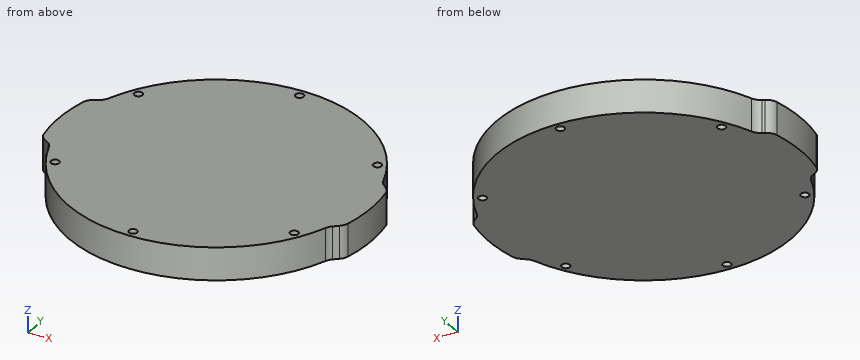
from build123d import *

# Parameters (mm, degrees)
SKETCH1_R           = 1.6
BOSS_EXTRUDE1_DEPTH = 12.7
FILLET1_R           = 5


with BuildPart() as part:
    # Sketch1 → Boss-Extrude1 (new body)
    with BuildSketch(Plane.XY):
        with BuildLine():
            Line((-59.281721466, 15), (-54.404710274, 17.5))
            ThreePointArc((-54.404710274, 17.5), (0, 57.15), (54.404710274, 17.5))
            Line((54.404710274, 17.5), (58.525108251, 13.886475587))
            ThreePointArc((58.525108251, 13.886475587), (60.15, 0), (58.525108251, -13.886475587))
            Line((58.525108251, -13.886475587), (54.404710274, -17.5))
            ThreePointArc((54.404710274, -17.5), (0, -57.15), (-54.404710274, -17.5))
            Line((-54.404710274, -17.5), (-59.281721466, -15))
            ThreePointArc((-59.281721466, -15), (-61.15, 0), (-59.281721466, 15))
        make_face()
        with Locations((0, 53.975)):
            Circle(SKETCH1_R, mode=Mode.SUBTRACT)
        with Locations((46.743721169, 26.9875)):
            Circle(SKETCH1_R, mode=Mode.SUBTRACT)
        with Locations((46.743721169, -26.9875)):
            Circle(SKETCH1_R, mode=Mode.SUBTRACT)
        with Locations((0, -53.975)):
            Circle(SKETCH1_R, mode=Mode.SUBTRACT)
        with Locations((-46.743721169, -26.9875)):
            Circle(SKETCH1_R, mode=Mode.SUBTRACT)
        with Locations((-46.743721169, 26.9875)):
            Circle(SKETCH1_R, mode=Mode.SUBTRACT)
    extrude(amount=BOSS_EXTRUDE1_DEPTH)

    # Fillet1
    fillet1_edges = [part.edges().sort_by_distance(p)[0] for p in [
        (58.525108251, -13.886475587, 6.35),
        (54.404710274, -17.5, 6.35),
        (-54.404710274, -17.5, 6.35),
        (-59.281721466, -15, 6.35),
        (-59.281721466, 15, 6.35),
        (-54.404710274, 17.5, 6.35),
        (54.404710274, 17.5, 6.35),
        (58.525108251, 13.886475587, 6.35),
    ]]
    fillet(fillet1_edges, radius=FILLET1_R)


solid = part.part
Read the model definition and answer for the solid it produces. Units are mm, in the model's axes. Coordinates: 2 decimals unless noted, no trailing zeros. Write each loop counter-clockwise with the first axis right and the second up, starting at its lowest first coordinate (ties: lowest second). Pieces come first, ordered by that corner, then holes. Notation, with made-up numbers: M 72,7.25 L 115,7.25 A8 cw 115,22.25 Z; hole C -23,86 d10. An arc over 180 degrees is marked long. Use a Markdown table: item, result.
Q1. The part is cut by section A-A, the plane x = 0. Write down the section's boundary in (y, z) (3 decimals).
Answer block:
| item | result |
|---|---|
| outline | M -57.15,0 L -55.575,0 L -55.575,12.7 L -57.15,12.7 Z; M -52.375,0 L 52.375,0 L 52.375,12.7 L -52.375,12.7 Z; M 55.575,0 L 57.15,0 L 57.15,12.7 L 55.575,12.7 Z |
Q2. The part is cut by section B-B, the plane z = 6.75. Give the number of separate pieces and of enclosed holes in the cut face, then the cut area to 3 significant figures.
Answer block:
| item | result |
|---|---|
| separate pieces | 1 |
| enclosed holes | 6 |
| area | 10,400 mm2 |
Q3. The part is cut by section C-C, the plane x = -47. Write down the section's boundary in (y, z), then the cut area to 3 significant figures.
Answer block:
| item | result |
|---|---|
| outline | M -32.51,0 L -28.57,0 L -28.57,12.7 L -32.51,12.7 Z; M -25.41,0 L 25.41,0 L 25.41,12.7 L -25.41,12.7 Z; M 28.57,0 L 32.51,0 L 32.51,12.7 L 28.57,12.7 Z |
| area | 746 mm2 |
Q4. Each of these flat-tipped pins is pushed along its axis until it touches: pin 1 Ø1.9 at (x, y) = (-46.74, 26.99) entering from +Z; pin 2 Ø3 at (y, z) = (34, 11) entering from +X; pin 3 Ø4 at (x, y) = (0, -53.975) entering from -Z; pin 4 Ø6 at (y, z) = (-19.5, 4.5) entering from -X. Where does it stop, or does it pass through?
Answer block:
| item | result |
|---|---|
| pin 1 | passes through |
| pin 2 | stops at x = 47.01 |
| pin 3 | stops at z = 0 |
| pin 4 | stops at x = -56.36 |
Q5. The part is cut by section D-D, the plane y = -32.5. Write down the section's boundary in (x, z), then the cut area to 3 significant figures.
Answer block:
| item | result |
|---|---|
| outline | M -47.01,0 L 47.01,0 L 47.01,12.7 L -47.01,12.7 Z |
| area | 1,190 mm2 |
Q6. Straight lines are drawn through the part: L1, parallel to X at y = -27, z = 6.25; L2, parallel to Y at x = -3, z = 8.5; L3, parallel to Y at x = 24, z = 8. For each, find the intervals that lie inside material, in ascending order. Write a range as [from, to].
Answer block:
| item | result |
|---|---|
| L1 | x = [-50.37, -48.34], [-45.14, 45.14], [48.34, 50.37] |
| L2 | y = [-57.07, 57.07] |
| L3 | y = [-51.87, 51.87] |
